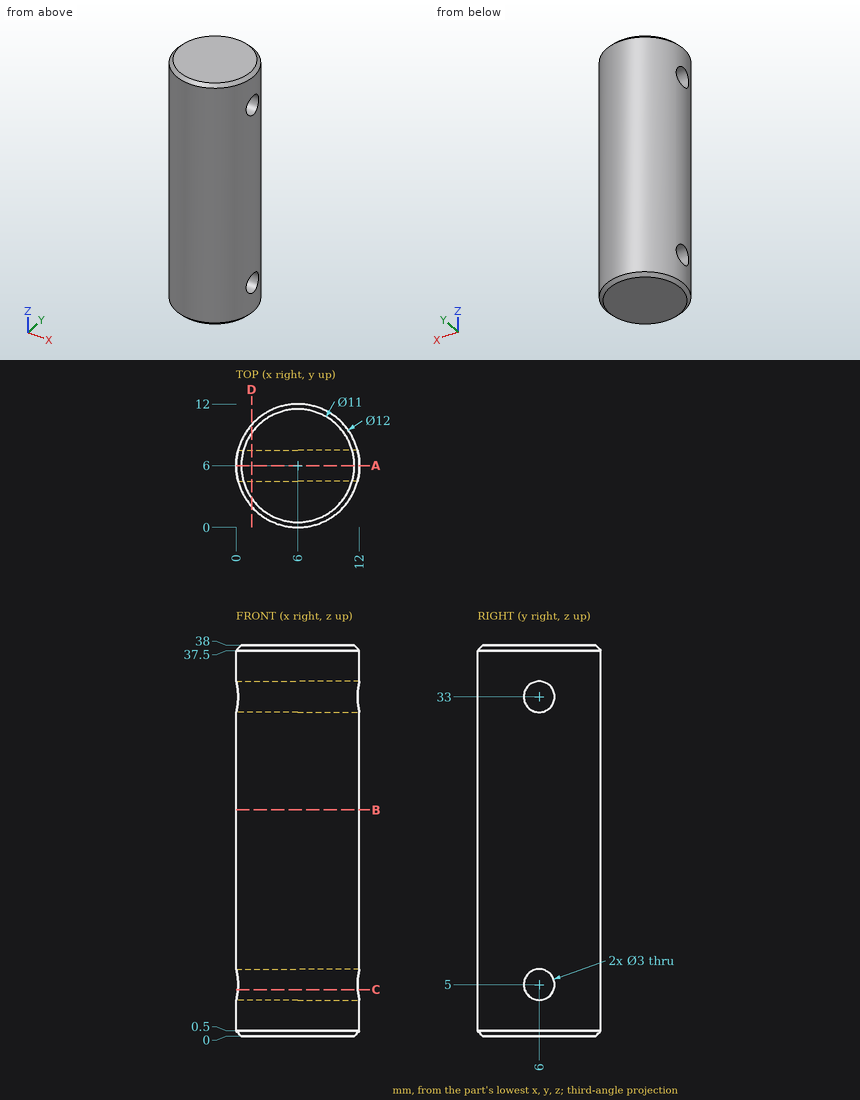
Could you check a few things on this drawing? It's one solid part, dimensions in mm from its lowest x, y, z. Round coordinates to 2 decimals unless told otherwise and drop trailing zeros. Write each loop counter-clockwise with the first axis right and the second up, starting at its lowest first coordinate (ties: lowest second). Pieces come first, ordered by that corner, then holes.
Q1. If we section it at B-B on z = 22: Write out the boundary of the cut face in (x, y).
Q2. If we section it at A-A on y = 6: Write out the boundary of the cut face in (x, z), plus the area to 4 significant figures.
Q3. Will these pins go through, and if not, where does the flat tip stop? P1, Ø1.5, axis at x = 3, z = 18, coming from the +Y side; P2, Ø1.5, axis at y = 8.5, z = 24.5, coming from the -X side.
Q4. If we section it at C-C on z = 4.5: Write out the boundary of the cut face in (x, y), plus the area to 3 significant figures.
Q5. Please list where these lines run through material, in increasing order: probe 1 along Z at (x, y) = (5.25, 7.25); probe 2 along Z at (x, y) = (11.5, 6.5); probe 3 along Y at (x, z) = (7.5, 5).
Q6. If we section it at D-D on x = 1.5: Give the number of separate pieces and of enclosed holes in the cut face, plus the area to 3 significant figures.
Answer below:
1. outline: circle Ø12 at (6, 6)
2. outline: (0, 0.5) - (0.5, 0) - (11.5, 0) - (12, 0.5) - (12, 3.5) - (0, 3.5) - close; (0, 6.5) - (12, 6.5) - (12, 31.5) - (0, 31.5) - close; (0, 34.5) - (12, 34.5) - (12, 37.5) - (11.5, 38) - (0.5, 38) - (0, 37.5) - close
2. area: 383.5 mm2
3. P1: stops at y = 11.56
3. P2: stops at x = 0.26
4. outline: (0.17, 4.59) arc R6 ccw to (11.83, 4.59) - close; (0.17, 7.41) - (11.83, 7.41) arc R6 ccw to start
4. area: 79.5 mm2
5. probe 1: z = 0 to 4.17, 5.83 to 32.17, 33.83 to 38
5. probe 2: z = 0.02 to 3.59, 6.41 to 31.59, 34.41 to 37.98
5. probe 3: y = 0.19 to 4.5, 7.5 to 11.81
6. separate pieces: 1
6. enclosed holes: 2
6. area: 287 mm2
